The drawing under review shows one solid part. Ordinate dimensions are in mm from its lowest x, y, z. Coordinates: 2 decimals unless noted, no trailing zeros. Loops run counter-clockwise (first coordinate to the right, second up) from the corner with the lowest first, then second, coordinate; pieces in that order, holes last. Notation, with made-up numbers: M 61.25,-36.75 L 118.25,-36.75 A33 cw 118.25,-2.75 Z; hole C 53.25,27.25 d10. An arc over 180 degrees is marked long. Answer as a JSON object with one key per item and string values. Group by question number.
1. Consider section B-B (x = 1.5). State the section outline as (y, z) points, then the cut area to 3 significant figures.
2. Insertion check: pin 1 (0.9 mm diameter, centred on y = 2.5, z = 21.5, fed in from +X); pin 2 (0.9 mm diameter, centred on y = 3, z = 21.5, fed in from -X); pin 3 (0.9 mm diameter, centred on x = 14, y = 2.5, fed in from +Z). Each pin has a flat end and moves straight along its axis. Give the tip position at first contact, or say it passes through.
3. Consider section C-C (y = 3.05). State the section outline as (x, z) points.
4. Consider section A-A (z = 33). State the section outline as (x, y) points, then the cut area to 3 significant figures.
5. To check wall thickness, follow probe 1 along Z at (x, y) = (9.25, 1.9); probe 2 along X at (y, z) = (2.95, 20). State the ranges of each line that lie inside material, in increasing order.
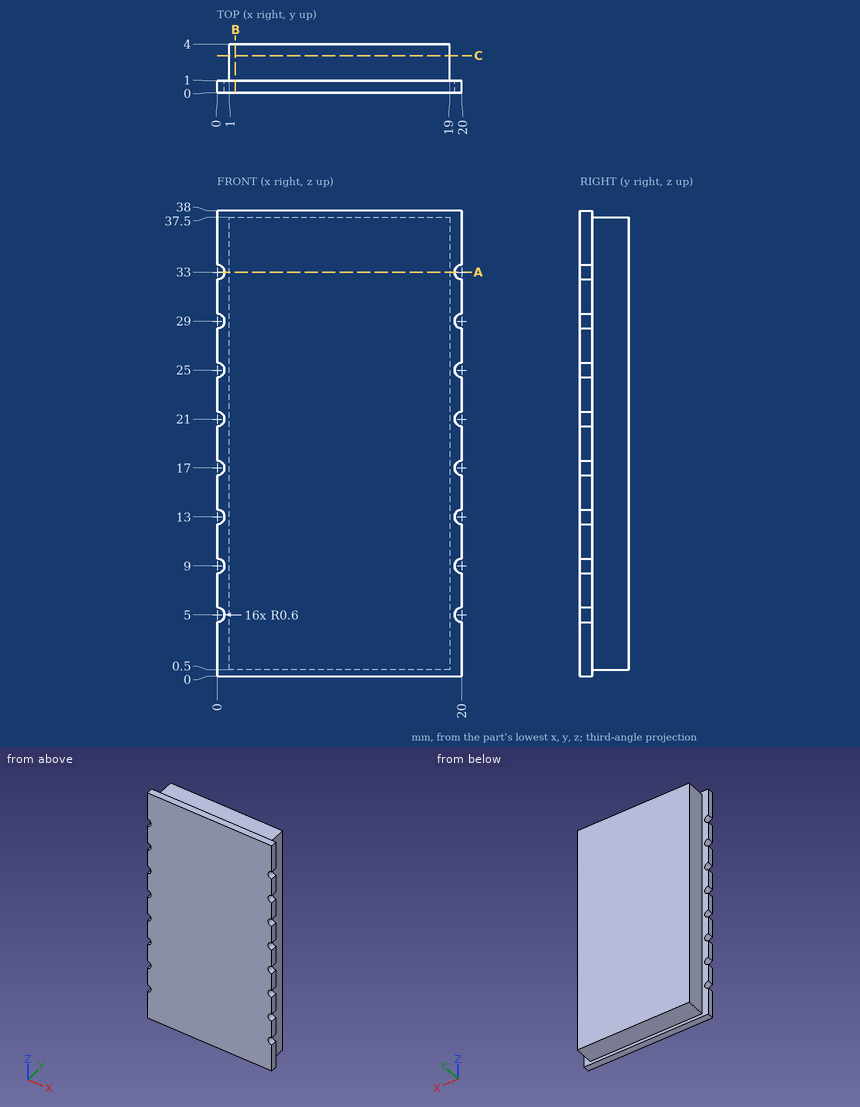
Findings below:
{
 "1": {"outline": "M 0,0 L 1,0 L 1,0.5 L 4,0.5 L 4,37.5 L 1,37.5 L 1,38 L 0,38 Z", "area": "149 mm^2"},
 "2": {"pin 1": "stops at x = 19", "pin 2": "stops at x = 1", "pin 3": "stops at z = 37.5"},
 "3": {"outline": "M 1,0.5 L 19,0.5 L 19,37.5 L 1,37.5 Z"},
 "4": {"outline": "M 0.6,0 L 19.4,0 L 19.4,1 L 19,1 L 19,4 L 1,4 L 1,1 L 0.6,1 Z", "area": "72.8 mm^2"},
 "5": {"probe 1": "z = 0.5 to 37.5", "probe 2": "x = 1 to 19"}
}
